Answer from the drawing. Dimensions are ordinates in mm from the lowest x, y and z of the part. A direction names the side the tool comes from. Round coordinates to 2 decimals unless told otherwise and drop trailing zeros. Write each loop counter-clockwise with the first axis right and the second up, starting at its lowest first coordinate (ties: lowest second). Pieces come first, ordered by that corner, then holes. Notation, with made-up numbers: M 58,-0.5 L 114,-0.5 A18 cw 114,15.5 Z; hole C 17,-22.5 d9. An arc over 180 degrees is marked long. One line per item, written item: value. Start each with the question number.
(1) Given P1, Ø1.5, axis at x = 5.5, z = 11.5, coming from the +Y side; P2, Ø3, axis at x = 6, y = 23.5, coming from the +Z side, each flat-ended and moving along its own axis, determine where each tip first touches the part or whether it passes through.
(2) Section A-A (z = 22.5) is taken. Determine the outline of the cut face in (x, y), plus the area to 3 significant figures.
(3) For a pull along X with two mould halves and no side action, classify the marked faces 3, 4 and 5 as released by +X, released by -X, zero draft, split by the parting line, or undercut.
(4) Section D-D (x = 7.5) is taken. Determine the outline of the cut face in (y, z), plus the area to 3 significant figures.
(5) Consider probe 1 along Y at (x, z) = (5.75, 18); probe 2 along X at (y, z) = (3.1, 22.5). Determine where each line is inside the solid, lowest interval first.
(6) For the marked faces 1 and 2, determine the directions among +Z, -Z, +X, -X, +Y, -Y from which every point of the face is accessible in a straight line to the end or side of a thin tool.
(7) Section B-B (x = 5) is taken. Determine the outline of the cut face in (y, z), plus the area to 3 significant figures.
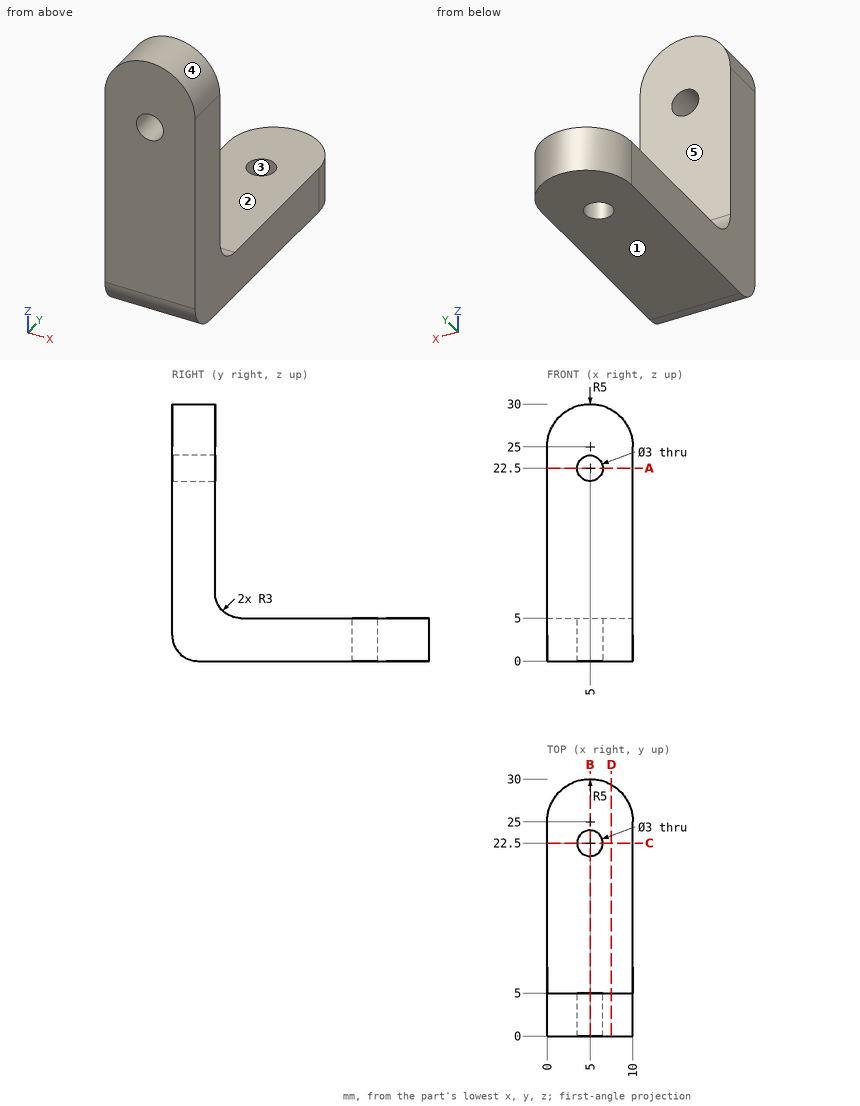
Recorded:
1. P1: stops at y = 5
1. P2: stops at z = 5
2. outline: M 0,0 L 3.5,0 L 3.5,5 L 0,5 Z; M 6.5,0 L 10,0 L 10,5 L 6.5,5 Z
2. area: 35.0 mm2
3. face 3: undercut
3. face 4: split by the parting line
3. face 5: zero draft
4. outline: M 0,3 A3 ccw 3,0 L 29.33,0 L 29.33,5 L 8,5 A3 cw 5,8 L 5,29.33 L 0,29.33 Z
4. area: 268 mm2
5. probe 1: y = 0 to 5
5. probe 2: x = 0 to 3.5, 6.5 to 10
6. face 1: -Z, +X, -X, +Y, -Y
6. face 2: +Z, +X, -X, +Y
7. outline: M 0,3 A3 ccw 3,0 L 21,0 L 21,5 L 8,5 A3 cw 5,8 L 5,21 L 0,21 Z; M 0,24 L 5,24 L 5,30 L 0,30 Z; M 24,0 L 30,0 L 30,5 L 24,5 Z
7. area: 245 mm2
